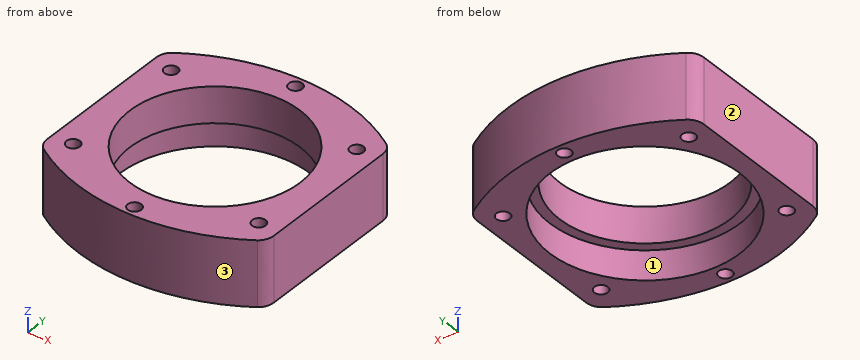
Autodesk Inventor part; units mm, degrees
ref_plane "YZ Plane" through (0, 0, 0) normal (1, 0, 0) x (0, 1, 0)
ref_plane "XZ Plane" through (0, 0, 0) normal (0, 1, 0) x (-1, 0, 0)
ref_plane "XY Plane" through (0, 0, 0) normal (0, 0, 1) x (1, 0, 0)
sketch "Sketch1" plane through (0, 0, 0) normal (0, 0, 1) x (1, 0, 0)
  circle A0 centre (28.6703, -20.0752) radius 2.067
  circle A1 centre (-28.6703, 20.0752) radius 2.067
  circle A2 centre (-28.6703, -20.0752) radius 2.067
  circle A3 centre (28.6703, 20.0752) radius 2.067
  circle A4 centre (0, 33) radius 2.067
  circle A5 centre (0, -33) radius 2.067
  spline S0 degree 3 poles (-33.0232, -26.3606) (-33.4707, -26.0209) (-33.8582, -25.6078) (-34.4385, -24.7312) (-34.6469, -24.2869) (-34.9285, -23.3518) (-35, -22.866) (-35, -22.3776) knots 0.026434 0.026434 0.026434 0.026434 0.19535 0.19535 0.341801 0.341801 0.488319 0.488319 0.488319 0.488319
  arc A6 (-33.0232, -26.3606) -> (33.0232, -26.3606) centre (0, 23.734) ccw
  spline S1 degree 3 poles (35, -22.3776) (35, -23.0287) (34.8729, -23.6735) (34.4404, -24.7277) (34.1898, -25.15) (33.6298, -25.8399) (33.3414, -26.119) (33.0232, -26.3606) knots 0 0 0 0 0.195306 0.195306 0.341836 0.341836 0.461894 0.461894 0.461894 0.461894
  line L0 (35, -22.3776) -> (35, 22.3638)
  spline S2 degree 3 poles (32.722, 26.5579) (33.2681, 26.2035) (33.7398, 25.7458) (34.3984, 24.7948) (34.6216, 24.3377) (34.9233, 23.3723) (35, 22.8695) (35, 22.3638) knots 0 0 0 0 0.195321 0.195321 0.347039 0.347039 0.498754 0.498754 0.498754 0.498754
  spline S3 degree 3 poles (32.6565, 26.6005) (32.6783, 26.5863) (32.7001, 26.5721) (32.722, 26.5579) knots 0 0 0 0 0.007808 0.007808 0.007808 0.007808
  arc A7 (32.6565, 26.6005) -> (-32.6565, 26.6005) centre (0, -23.734) ccw
  spline S4 degree 3 poles (-32.6565, 26.6005) (-32.6783, 26.5863) (-32.7001, 26.5721) (-32.722, 26.5579) knots -3.47 -3.47 -3.47 -3.47 -3.462013 -3.462013 -3.462013 -3.462013
  spline S5 degree 3 poles (-35, 22.3638) (-35, 23.0149) (-34.8728, 23.6598) (-34.4336, 24.7299) (-34.1718, 25.166) (-33.5262, 25.9446) (-33.1462, 26.2826) (-32.722, 26.5579) knots 0 0 0 0 0.195326 0.195326 0.347039 0.347039 0.498754 0.498754 0.498754 0.498754
  line L1 (-35, 22.3638) -> (-35, -22.3776)
  circle A8 centre (0, 0) radius 26.25
  dimension "d2" = 33
  dimension "d3" = 33
extrude "Extrusion1" add sketch "Sketch1" along normal blind 20
sketch "Sketch2" plane through (0, 0, 0) normal (0, 0, -1) x (-1, 0, 0)
  circle A0 centre (0, 0) radius 29.2625
  dimension "d4" = 58.525
extrude "Extrusion2" cut sketch "Sketch2" against normal blind 9
properties part number "Tilting head - extended part" material "Steel, Carbon"
For this review, take the finished solid that the model builds, in its own axes (mm). Face numbers are marked on the shaded views. Give positions to 0.01 mm unless a question says otherwise; leave off trailing zeros. Order: outer loops, then holes, each group sorted by start corner. A loop starts at its lowest first (then second) coordinate and runs counter-clockwise, first axis right, second up.
1) Take a section at D-D (y = -33). Give the boundary of the cut face in (x, z), then the cut area to 3 significant figures.
2) The part is to be moulded in two halves that separate along Y. For the marked faces 1, 2 and 3, say which applies: released by +Y, released by -Y, zero draft, split by the parting line, or undercut.
3) Wall thickness on line 1 (Y direction, x = 0.5, z = 15.5); line 2 (X direction, y = 0, z = 17); line 3 (X direction, y = 21, z = 6.5): over which ranges is each line inside the solid? List them lowest first.
4) Take a section at C-C (x = -25). Give the boundary of the cut face in (y, z).
5) Take a section at B-B (y = 0). Give the boundary of the cut face in (x, z).
6) Insertion check: pin 1 (4 mm diameter, centred on x = 6, z = 4.5, fed in from +Y); pin 2 (2 mm diameter, centred on x = -8, z = 3, fed in from +Y); pin 3 (3.5 mm diameter, centred on x = 28.67, y = -20.08, fed in from +Z); pin 4 (8 mm diameter, centred on x = -9, z = 9, fed in from -Y). Each pin has a flat end and moves straight along its axis. Give the tip position at first contact, or say it passes through.
7) Take a section at A-A (x = 0). Give the boundary of the cut face in (y, z), then the cut area to 3 significant figures.
Derived:
1. outline: (-19.53, 0) - (-2.07, 0) - (-2.07, 20) - (-19.53, 20) - close; (2.07, 0) - (19.53, 0) - (19.53, 20) - (2.07, 20) - close
1. area: 698 mm2
2. face 1: undercut
2. face 2: zero draft
2. face 3: released by -Y
3. line 1: y = -36.26 to -35.01, -30.99 to -26.25, 26.25 to 30.99, 35.01 to 36.26
3. line 2: x = -35 to -26.25, 26.25 to 35
3. line 3: x = -35 to -30.52, -26.82 to -20.38, 20.38 to 26.82, 30.52 to 35
4. outline: (-30.81, 0) - (-15.21, 0) - (-15.21, 9) - (-8, 9) - (-8, 20) - (-30.81, 20) - close; (8, 9) - (15.21, 9) - (15.21, 0) - (30.81, 0) - (30.81, 20) - (8, 20) - close
5. outline: (-35, 0) - (-29.26, 0) - (-29.26, 9) - (-26.25, 9) - (-26.25, 20) - (-35, 20) - close; (26.25, 9) - (29.26, 9) - (29.26, 0) - (35, 0) - (35, 20) - (26.25, 20) - close
6. pin 1: stops at y = 36.13
6. pin 2: stops at y = 35.86
6. pin 3: passes through
6. pin 4: stops at y = -36.06
7. outline: (-36.27, 0) - (-35.07, 0) - (-35.07, 20) - (-36.27, 20) - close; (-30.93, 0) - (-29.26, 0) - (-29.26, 9) - (-26.25, 9) - (-26.25, 20) - (-30.93, 20) - close; (26.25, 9) - (29.26, 9) - (29.26, 0) - (30.93, 0) - (30.93, 20) - (26.25, 20) - close; (35.07, 0) - (36.27, 0) - (36.27, 20) - (35.07, 20) - close
7. area: 181 mm2
